Drawing for the job (mm, zero at the part's lowest x, y, z). Give positions to 0.01 mm unless a question says otherwise; leave off trailing zeros. Write each loop counter-clockwise with the first axis right and the second up, starting at its lowest first coordinate (ties: lowest second). Pieces come first, ordered by that corner, then holes. Notation, with made-up numbers: M -24.5,21.5 L 32.5,21.5 A31 cw 32.5,49.5 Z; hole C 68.5,46 d11. An arc over 180 degrees is marked long. Write item = value, one per line. Start each with the question number.
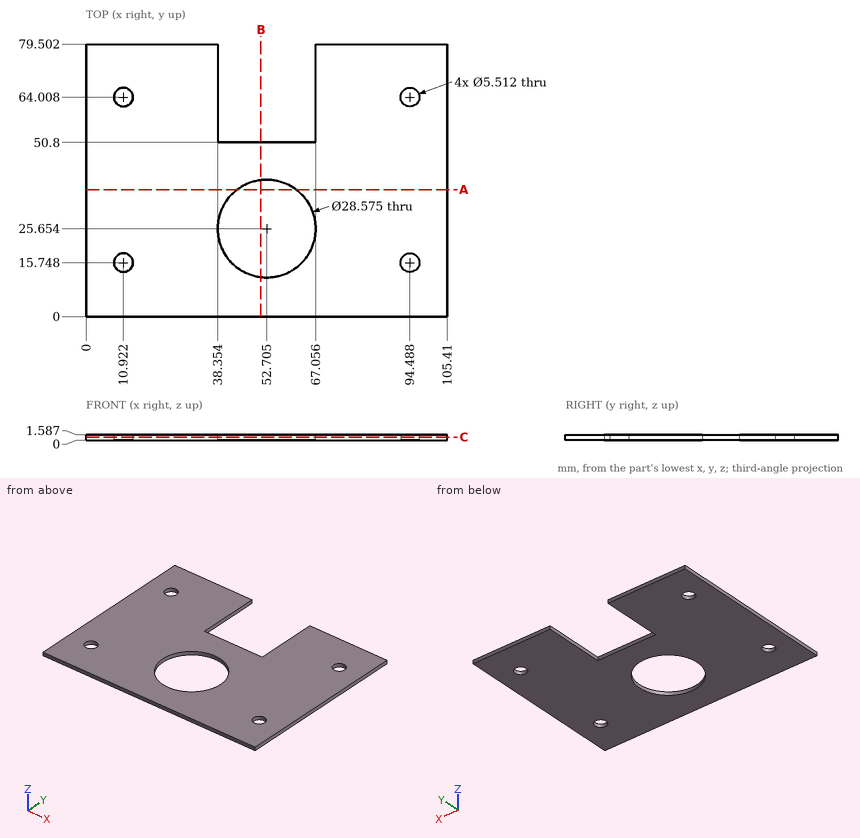
Q1. Slice it at B-B (x = 51). Give the cut face in (y, z).
Q2. Slice it at C-C (z = 0.85). Give the cut face in (x, y) (1 decimal), and give its area (3 significant figures).
Q3. Drop flat-ended pins along their axis: P1, Ø7, axis at x = 10.922, y = 15.748, coming from the -Z side; P2, Ø0.5, axis at x = 54.5, z = 1, coming from the +Y side. Give the stop position or say it passes through.
Q4. Slice it at A-A (y = 37). Give the cut face in (x, z).
Q5. Probe line 1 along X through (y, z) = (57, 1.35) (1 decimal); line 2 along Y through (x, z) = (96.5, 0.45) (1 decimal); line 3 along X through (y, z) = (18, 1.1) (1 decimal). List the from-to ranges inside material, lowest first.
Working result:
q1.outline = M 0,0 L 11.47,0 L 11.47,1.59 L 0,1.59 Z; M 39.84,0 L 50.8,0 L 50.8,1.59 L 39.84,1.59 Z
q2.outline = M 0,0 L 105.4,0 L 105.4,79.5 L 67.1,79.5 L 67.1,50.8 L 38.4,50.8 L 38.4,79.5 L 0,79.5 Z; hole C 10.9,15.7 d5.5; hole C 10.9,64 d5.5; hole C 52.7,25.7 d28.6; hole C 94.5,15.7 d5.5; hole C 94.5,64 d5.5
q2.area = 6,820 mm2
q3.P1 = 0
q3.P2 = 50.8
q4.outline = M 0,0 L 44.02,0 L 44.02,1.59 L 0,1.59 Z; M 61.39,0 L 105.41,0 L 105.41,1.59 L 61.39,1.59 Z
q5.line_1 = 0 to 38.4, 67.1 to 105.4
q5.line_2 = 0 to 13.9, 17.6 to 62.1, 65.9 to 79.5
q5.line_3 = 0 to 9.3, 12.5 to 40.6, 64.8 to 92.9, 96.1 to 105.4
